Can you work these out from the model? Positions are in its coordinate system, mm. Coordinates: 2 decimals unless noted, no trailing zeros. Loops run counter-clockwise (first coordinate to the right, second up) from the corner with the lowest first, then second, coordinate; pieces in that order, holes last. Notation, with made-up numbers: (-23.5, 79) -> (20.5, 79) arc R24 cw to (20.5, 112) -> close; hole circle Ø1 at (86, 34). An arc over 180 degrees is marked (long way). Put each result on its own line as item: value. Start each with the question number.
Item 1: If we section it at A-A on x = 19: Please give me the cut outline in (y, z) (1 decimal), plus the area to 3 significant figures.
Item 2: Please list where these lines run through material, in increasing order: L1, parallel to X at y = 41, z = 3.05; L2, parallel to Y at x = 28, z = 2.8; L3, parallel to Y at x = 25.4, z = 0.75. Write a range as from..to.
Item 3: Will this pin go through, and if not, where does the flat tip stop? P1, Ø4, axis at x = 25.4, y = 21.78, coming from the +Z side.
Item 4: If we section it at D-D on y = 42: Please give me the cut outline in (x, z) (3 decimals), plus the area to 3 significant figures.
Item 5: If we section it at B-B on y = 127.5: Please give me the cut outline in (x, z) (3 decimals), plus the area to 3 significant figures.
Item 6: If we section it at C-C on z = 0.85: State how many separate pieces and enclosed holes the cut face has, plus the area to 3 significant figures.
```python
from build123d import *

# Parameters (mm, degrees)
SKETCH1_W           = 31.75
SKETCH1_H           = 147.32
BOSS_EXTRUDE1_DEPTH = 3.175
CUT_EXTRUDE4_REACH  = 5.175
SKETCH5_W           = 31.75
SKETCH5_H           = 5.842
CUT_EXTRUDE5_REACH  = 5.175
SKETCH6_W           = 31.75
SKETCH6_H           = 0.0635
CUT_EXTRUDE6_REACH  = 5.175
SKETCH8_R           = 3.175
SKETCH10_R          = 9.525
CUT_EXTRUDE7_DEPTH  = 4.175


with BuildPart() as part:
    # Sketch1 → Boss-Extrude1 (new body)
    with BuildSketch(Plane.XY):
        with Locations((15.875, 73.66)):
            Rectangle(SKETCH1_W, SKETCH1_H)
    extrude(amount=BOSS_EXTRUDE1_DEPTH)

    # Sketch5 → Cut-Extrude4 (cut, up to next)
    with BuildSketch(Plane.XY.offset(3.175), mode=Mode.PRIVATE) as cut_extrude4_sk1:
        with Locations((15.875, 2.921)):
            Rectangle(SKETCH5_W, SKETCH5_H)
    cut_extrude4_tool1 = extrude(cut_extrude4_sk1.sketch, amount=-CUT_EXTRUDE4_REACH, mode=Mode.PRIVATE) & part.part
    add(cut_extrude4_tool1.solids().sort_by_distance((15.875, 2.921, 3.175))[0], mode=Mode.SUBTRACT)

    # Sketch6 → Cut-Extrude5 (cut, up to next)
    with BuildSketch(Plane.XY.offset(3.175), mode=Mode.PRIVATE) as cut_extrude5_sk1:
        with Locations((15.875, 5.87375)):
            Rectangle(SKETCH6_W, SKETCH6_H)
    cut_extrude5_tool1 = extrude(cut_extrude5_sk1.sketch, amount=-CUT_EXTRUDE5_REACH, mode=Mode.PRIVATE) & part.part
    add(cut_extrude5_tool1.solids().sort_by_distance((15.875, 5.87375, 3.175))[0], mode=Mode.SUBTRACT)

    # Sketch8 → Cut-Extrude6 (cut, up to next)
    with BuildSketch(Plane.XY.offset(3.175), mode=Mode.PRIVATE) as cut_extrude6_sk1:
        with Locations((25.4, 40.8305)):
            Circle(SKETCH8_R)
    cut_extrude6_tool1 = extrude(cut_extrude6_sk1.sketch, amount=-CUT_EXTRUDE6_REACH, mode=Mode.PRIVATE) & part.part
    add(cut_extrude6_tool1.solids().sort_by_distance((25.4, 40.8305, 3.175))[0], mode=Mode.SUBTRACT)
    # Sketch8 → Cut-Extrude6 (cut, up to next)
    with BuildSketch(Plane.XY.offset(3.175), mode=Mode.PRIVATE) as cut_extrude6_sk2:
        with Locations((6.35, 40.8305)):
            Circle(SKETCH8_R)
    cut_extrude6_tool2 = extrude(cut_extrude6_sk2.sketch, amount=-CUT_EXTRUDE6_REACH, mode=Mode.PRIVATE) & part.part
    add(cut_extrude6_tool2.solids().sort_by_distance((6.35, 40.8305, 3.175))[0], mode=Mode.SUBTRACT)
    # Sketch8 → Cut-Extrude6 (cut, up to next)
    with BuildSketch(Plane.XY.offset(3.175), mode=Mode.PRIVATE) as cut_extrude6_sk3:
        with Locations((6.35, 21.7805)):
            Circle(SKETCH8_R)
    cut_extrude6_tool3 = extrude(cut_extrude6_sk3.sketch, amount=-CUT_EXTRUDE6_REACH, mode=Mode.PRIVATE) & part.part
    add(cut_extrude6_tool3.solids().sort_by_distance((6.35, 21.7805, 3.175))[0], mode=Mode.SUBTRACT)
    # Sketch8 → Cut-Extrude6 (cut, up to next)
    with BuildSketch(Plane.XY.offset(3.175), mode=Mode.PRIVATE) as cut_extrude6_sk4:
        with Locations((25.4, 21.7805)):
            Circle(SKETCH8_R)
    cut_extrude6_tool4 = extrude(cut_extrude6_sk4.sketch, amount=-CUT_EXTRUDE6_REACH, mode=Mode.PRIVATE) & part.part
    add(cut_extrude6_tool4.solids().sort_by_distance((25.4, 21.7805, 3.175))[0], mode=Mode.SUBTRACT)

    # Sketch10 → Cut-Extrude7 (cut, through all)
    with BuildSketch(Plane.XY.offset(3.175)):
        with Locations((15.7861, 131.5339)):
            Circle(SKETCH10_R)
        with BuildLine():
            ThreePointArc((6.5786, 120.5738), (4.826, 122.3264), (3.0734, 120.5738))
            ThreePointArc((3.0734, 120.5738), (4.826, 118.8212), (6.5786, 120.5738))
        make_face()
        with BuildLine():
            ThreePointArc((24.9936, 142.494), (26.7462, 140.7414), (28.4988, 142.494))
            ThreePointArc((28.4988, 142.494), (26.7462, 144.2466), (24.9936, 142.494))
        make_face()
    extrude(amount=-CUT_EXTRUDE7_DEPTH, mode=Mode.SUBTRACT)


solid = part.part
```
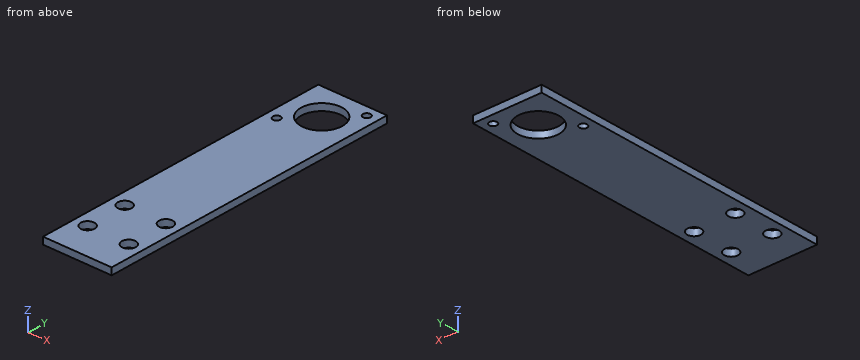
Solutions:
1. outline: (5.9, 0) -> (122.6, 0) -> (122.6, 3.2) -> (5.9, 3.2) -> close; (140.5, 0) -> (147.3, 0) -> (147.3, 3.2) -> (140.5, 3.2) -> close
1. area: 392 mm^2
2. L1: 0..3.18, 9.52..22.23, 28.57..31.75
2. L2: 5.91..19.96, 23.6..39.01, 42.65..141.27, 143.72..147.32
2. L3: 5.91..18.61, 24.96..37.66, 44.01..141.37, 143.62..147.32
3. P1: through
4. outline: (0, 0) -> (3.398, 0) -> (3.398, 3.175) -> (0, 3.175) -> close; (9.302, 0) -> (22.448, 0) -> (22.448, 3.175) -> (9.302, 3.175) -> close; (28.352, 0) -> (31.75, 0) -> (31.75, 3.175) -> (28.352, 3.175) -> close
4. area: 63.3 mm^2
5. outline: (0, 0) -> (7.157, 0) -> (7.157, 3.175) -> (0, 3.175) -> close; (24.415, 0) -> (31.75, 0) -> (31.75, 3.175) -> (24.415, 3.175) -> close
5. area: 46.0 mm^2
6. separate pieces: 1
6. enclosed holes: 7
6. area: 4,060 mm^2
